CAD build for the part. Positions are in the model's coordinates, mm. Face numbers are marked on the shaded views. A direction names the side the tool comes from. Round coordinates to 2 decimals unless told otherwise and drop trailing zeros. Order: outer loops, then holes, each group sorted by start corner. A loop starts at its lowest first (then second) coordinate and runs counter-clockwise, first axis right, second up. Notation, with made-up numbers: M -19,-28.5 L -12,-28.5 A26 cw -12,-12.5 Z; hole C -29,-2 d10. An arc over 180 degrees is marked long. Answer as a JSON object with one key per item and string values. Group by question number.
```python
from build123d import *

# Parameters (mm, degrees)
SCHIZZO1_W                   = 28
SCHIZZO1_H                   = 22
ESTRUSIONE_ESTRUSIONE1_DEPTH = 9
SCHIZZO2_W                   = 24
SCHIZZO2_H                   = 13
ESTRUSIONE_ESTRUSIONE2_DEPTH = 8.4
SCHIZZO3_R                   = 6.5
SCHIZZO3_R_2                 = 5.5
ESTRUSIONE_ESTRUSIONE3_DEPTH = 1
SCHIZZO5_OUTSIDE_W           = 38.016
SCHIZZO5_OUTSIDE_H           = 32.016
SCHIZZO5_OUTSIDE_R           = 12
TAGLIO_ESTRUSIONE1_DEPTH     = 10
SCHIZZO6_W                   = 28
SCHIZZO6_H                   = 22
TAGLIO_ESTRUSIONE2_DEPTH     = 14
SCHIZZO7_R                   = 1.5
ESTRUSIONE_ESTRUSIONE4_DEPTH = 5
ESTRUSIONE_ESTRUSIONE5_DEPTH = 9
TAGLIO_ESTRUSIONE3_DEPTH     = 7
RIPETIZIONE_A_L1_COUNT       = 7
RIPETIZIONE_A_L1_PITCH       = 4


with BuildPart() as part:
    # Schizzo1 → Estrusione-Estrusione1 (new body)
    with BuildSketch(Plane(origin=(0, 0, 0), x_dir=(1, 0, 0), z_dir=(0, 1, 0))):
        Rectangle(SCHIZZO1_W, SCHIZZO1_H)
    extrude(amount=ESTRUSIONE_ESTRUSIONE1_DEPTH)

    # Schizzo2 → Estrusione-Estrusione2 (add)
    with BuildSketch(Plane(origin=(0, 9, 0), x_dir=(1, 0, 0), z_dir=(0, 1, 0))):
        Rectangle(SCHIZZO2_W, SCHIZZO2_H)
    extrude(amount=ESTRUSIONE_ESTRUSIONE2_DEPTH)

    # Schizzo3 → Estrusione-Estrusione3 (add)
    with BuildSketch(Plane(origin=(0, 17.4, 0), x_dir=(1, 0, 0), z_dir=(0, 1, 0))):
        with Locations(Location((0, 0, 0), (0, 0, 270))):
            Circle(SCHIZZO3_R)
        with Locations(Location((0, 0, 0), (0, 0, 270))):
            Circle(SCHIZZO3_R_2, mode=Mode.SUBTRACT)
    extrude(amount=ESTRUSIONE_ESTRUSIONE3_DEPTH)

    # Schizzo5 outside → Taglio-Estrusione1 (cut)
    with BuildSketch(Plane(origin=(0, 17.4, 0), x_dir=(1, 0, 0), z_dir=(0, 1, 0))):
        Rectangle(SCHIZZO5_OUTSIDE_W, SCHIZZO5_OUTSIDE_H)
        Circle(SCHIZZO5_OUTSIDE_R, mode=Mode.SUBTRACT)
    extrude(amount=-TAGLIO_ESTRUSIONE1_DEPTH, mode=Mode.SUBTRACT)

    # Schizzo6 → Taglio-Estrusione2 (cut)
    with BuildSketch(Plane.XZ):
        Rectangle(SCHIZZO6_W, SCHIZZO6_H)
    extrude(amount=-TAGLIO_ESTRUSIONE2_DEPTH, mode=Mode.SUBTRACT)

    # Schizzo7 → Estrusione-Estrusione4 (add)
    with BuildSketch(Plane.XZ.offset(-14)):
        with Locations(Location((-9.5, 0, 0), (0, 0, 90))):
            Circle(SCHIZZO7_R)
        with Locations(Location((9.5, 0, 0), (0, 0, 90))):
            Circle(SCHIZZO7_R)
    extrude(amount=ESTRUSIONE_ESTRUSIONE4_DEPTH)

    # Schizzo3D1 → Estrusione-Estrusione5 (add)
    with BuildSketch(Plane(origin=(14, 9, 11), x_dir=(-0.7863183388224227, 0, -0.6178215519319035), z_dir=(0, -1, 0))):
        Polygon((0, 0), (22.016913487, -17.299003454), (35.60898763, 0), (13.592074143, 17.299003454), align=None)
    extrude(amount=ESTRUSIONE_ESTRUSIONE5_DEPTH)

    # Schizzo3D2 → Taglio-Estrusione3 (cut)
    with BuildSketch(Plane(origin=(-13.5, 0, 11), x_dir=(0.13511320473331354, 0, -0.990830168044299), z_dir=(0, -1, 0))):
        Polygon((0, 0), (0.405339614, 2.972490504), (22.203603311, 0), (21.798263697, -2.972490504), align=None)
    taglio_estrusione3 = extrude(amount=-TAGLIO_ESTRUSIONE3_DEPTH, mode=Mode.SUBTRACT)

    # Ripetizione a L1: Taglio-Estrusione3 ×7
    with Locations(*[(i * RIPETIZIONE_A_L1_PITCH, 0, 0) for i in range(1, RIPETIZIONE_A_L1_COUNT)]):
        add(taglio_estrusione3, mode=Mode.SUBTRACT)


solid = part.part
```
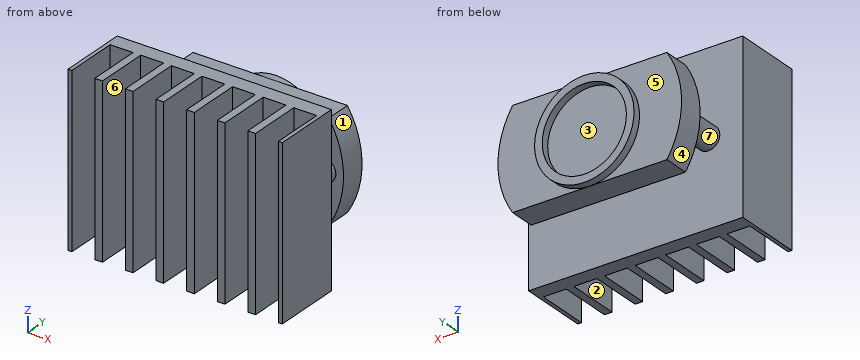
Item 1: Drill centre lines: line 1 (X direction, y = 18.25, z = 0); line 2 (Y direction, x = 8, z = 3.5); line 3 (Y direction, x = 12.75, z = 4). Where is each one in solid material? Low to high. Write a range as [from, to].
Item 2: Cut at D-D, the plane x = -8.5. Give the cut face in (y, z), and give its area (3 significant figures).
Item 3: Cut at A-A, the plane y = 1.5. Give the number of separate pieces and of enclosed holes in the cut face, and give its area (3 significant figures).
Item 4: Cut at C-C, the plane x = 3.25. Give the cut face in (y, z).
Item 5: Flat gauge pins, fed straight in: pin 1 Ø1.5 at (x, z) = (-8.5, 4) entering from -Y; pin 2 Ø10 at (x, z) = (0, 0) entering from +Y. Where does each tip first touch, or does it go through?
Item 6: 3-axis set-ups, long thin cutter, end or side, ignore diameter. For the marked faces 1, 2, 3 and 4: which of +Z, -Z, +X, -X, +Y, -Y reach the whole face in a straight line?
Item 7: Two-plate mould, pull along Y, no slides. Class the marked faces 5, 6 and 7: +Y half, -Y half, draft (parallel to the pull), parting line (faces both ways), or undercut.
Response values:
{
 "1": {"line 1": "[-6.5, -5.5], [5.5, 6.5]", "line 2": "[7, 9], [14, 17.4]", "line 3": "[7, 9]"},
 "2": {"outline": "M 7,-11 L 9,-11 L 9,-1.12 L 14,-1.12 L 14,-6.5 L 17.4,-6.5 L 17.4,6.5 L 14,6.5 L 14,1.12 L 9,1.12 L 9,11 L 7,11 Z", "area": "99.4 mm^2"},
 "3": {"separate pieces": "8", "enclosed holes": "0", "area": "154 mm^2"},
 "4": {"outline": "M 7,-11 L 9,-11 L 9,11 L 7,11 Z; M 14,-6.5 L 17.4,-6.5 L 17.4,-5.63 L 18.4,-5.63 L 18.4,-4.44 L 17.4,-4.44 L 17.4,4.44 L 18.4,4.44 L 18.4,5.63 L 17.4,5.63 L 17.4,6.5 L 14,6.5 Z"},
 "5": {"pin 1": "y = 7", "pin 2": "y = 17.4"},
 "6": {"face 1": "+X, +Y", "face 2": "+Z, -Z, -Y", "face 3": "+Y", "face 4": "-X, +Y"},
 "7": {"face 5": "+Y half", "face 6": "draft", "face 7": "undercut"}
}
